The model under review builds one solid part; all positions refer to its coordinate system, in mm. Face numbers are marked on the shaded views. A direction names the side the tool comes from. Give positions to 0.01 mm unless a question says otherwise; leave off trailing zeros. Order: outer loops, then holes, each group sorted by start corner. A loop starts at its lowest first (then second) coordinate and runs counter-clockwise, first axis right, second up. Notation, with made-up numbers: (55.5, 77.25) - (82.5, 77.25) arc R34 cw to (82.5, 114.25) - close; hole circle Ø4 at (28.5, 75). An arc over 180 degrees is marked (long way). Put each result on its own line as item: value.
Autodesk Inventor part; units mm, degrees
ref_plane "Work Plane1" through (-126.3, 142.5, 0) normal (0, 1, 0) x (-1, 0, 0)
ref_plane "Work Plane2" through (0, 0, 0) normal (0, 1, 0) x (-1, 0, 0)
ref_plane "Work Plane3" through (0, 0, 0) normal (0, 0, 1) x (1, 0, 0)
sketch "Sketch1" plane through (0, 0, 0) normal (0, 0, 1) x (1, 0, 0)
  line L0 (-126.3, 0) -> (126.3, 0)
  line L1 (126.3, 0) -> (126.3, 142.5)
  line L2 (126.3, 0) -> (268.8, 0) construction
  line L3 (-126.3, 0) -> (-126.3, 142.5)
  point P0 (0, 0)
  dimension "d0" = 252.6
  dimension "d1" = 142.5
  dimension "d2" = 90
  dimension "d3" = 142.5
ref_plane "Work Plane1" through (-126.3, 142.5, 0) normal (0, 1, 0) x (-1, 0, 0)
sketch "Sketch2" plane through (-126.3, 142.5, 0) normal (0, 1, 0) x (-1, 0, 0)
  circle A0 centre (0, 0) radius 10.65
  point P0 (-126.3, 0)
  dimension "d4" = 21.3
sweep "Sweep1" add profiles "Sketch2" path "Sketch1"
ref_plane "Work Plane2" through (0, 0, 0) normal (0, 1, 0) x (-1, 0, 0)
sketch "Sketch3" plane through (0, 0, 0) normal (0, 1, 0) x (-1, 0, 0)
  circle A0 centre (0, 0) radius 11
  dimension "d8" = 22
extrude "Extrusion1" add sketch "Sketch3" along normal blind 17.5
ref_plane "Work Plane3" through (0, 0, 0) normal (0, 0, 1) x (1, 0, 0)
sketch "Sketch4" plane through (0, 0, 0) normal (0, 0, 1) x (1, 0, 0)
  circle A0 centre (0, 12.5) radius 2.5
  point P0 (0, 0)
  dimension "d12" = 5
extrude "Extrusion2" cut sketch "Sketch4" along normal mid plane 100
ref_plane "Work Plane4" through (0, 0, 0) normal (1, 0, 0) x (0, 1, 0)
sketch "Sketch5" plane through (0, 0, 0) normal (1, 0, 0) x (0, 1, 0)
  circle A0 centre (12.5, 0) radius 2.5
  point P0 (0, 0)
  dimension "d16" = 5
extrude "Extrusion3" cut sketch "Sketch5" along normal mid plane 100
sketch "Sketch6" plane through (-126.3, 142.5, 0) normal (0, 1, 0) x (1, 0, 0)
  circle A0 centre (0, 0) radius 10.65
  point P0 (126.3, 0)
sketch "Sketch7" plane through (126.3, 142.5, 0) normal (0, 1, 0) x (1, 0, 0)
  circle A0 centre (0, 0) radius 10.65
  point P0 (-126.3, 0)
ref_plane "Work Plane6" through (126.3, 0, 0) normal (1, 0, 0) x (0, 1, 0)
ref_plane "Work Plane7" through (-126.3, 0, 0) normal (1, 0, 0) x (0, 1, 0)
sketch "Sketch8" plane through (-126.3, 0, 0) normal (1, 0, 0) x (0, 1, 0)
  line L0 (142.5, -10.65) -> (142.5, 10.65)
  circle A0 centre (130, 0) radius 10.65
  point P0 (0, 0)
  point P1 (142.5, 0)
  dimension "d21" = 21.3
extrude "Extrusion4" add sketch "Sketch8" against normal blind 100
sketch "Sketch9" plane through (126.3, 0, 0) normal (1, 0, 0) x (0, 1, 0)
  circle A0 centre (130, 0) radius 10.65
  circle A1 centre (130, 0) radius 10.65
  point P0 (0, 0)
extrude "Extrusion5" add sketch "Sketch9" along normal blind 100
properties part number "hands" material "PVC-Piping"
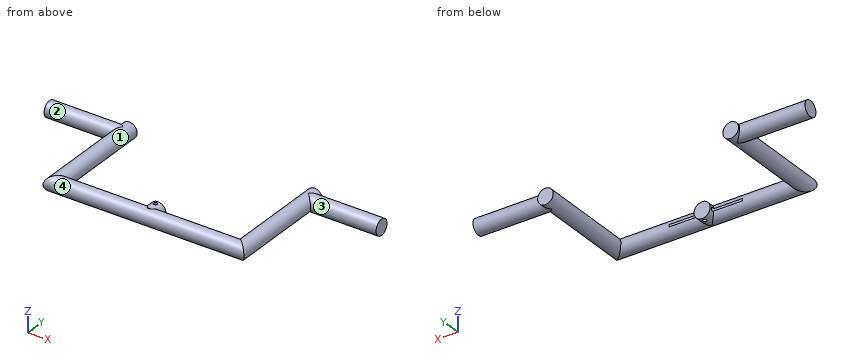
(1) Wall thickness on L1, parallel to X at y = 16.5, z = -1; L2, parallel to X at y = 42, z = 1; L3, parallel to X at y = 12.5, z = 2.75: over which ranges is each line inside the solid? List them lowest first.
The answers:
L1: -136.9 to -115.7, -10.95 to 10.95, 115.7 to 136.9
L2: -136.9 to -115.7, 115.7 to 136.9
L3: -136.59 to -116.01, -10.65 to -2.5, 2.5 to 10.65, 116.01 to 136.59
(2) Take a section at D-D, the plane x = -27. Write out the cut boundary in (y, z), then the cut area to 3 significant figures.
The answers:
outline: (10.54, -1.55) arc R2.5 cw to (10.54, 1.55) arc R10.65 ccw (long way) to start
area: 355 mm^2
(3) The part is to be moulded in two halves that separate along X. For the marked faces 3 and 4, say which applies: pulls with the +X half, pulls with the -X half, needs draft (parallel to the pull), parting line crosses it, or undercut.
The answers:
face 3: needs draft
face 4: undercut
(4) Take a section at B-B, the plane x = 130.5. Write out the cut boundary in (y, z), then the cut area to 3 significant figures.
The answers:
outline: (-4.2, -9.79) - (125.8, -9.79) arc R10.65 ccw to (134.2, -9.79) - (142.5, -9.79) - (142.5, 9.79) - (134.2, 9.79) arc R10.65 ccw to (125.8, 9.79) - (-4.2, 9.79) arc R10.65 ccw to start
area: 2,970 mm^2
(5) For the marked faces 1 and 2, list the 3-axis set-ups (+Z, -Z, +X, -X, +Y, -Y) from which the entire face can be reached by the end or side of a thin tool; tool diameter is ignored.
The answers:
face 1: none
face 2: -X
(6) Clearance check with flat-ended pins moving along their axes: pin 1 Ø5 at (x, z) = (179.5, 7) entering from -Y; pin 2 Ø8 at (y, z) = (69.5, 4) entering from +X; pin 3 Ø2 at (x, z) = (-92, 4.5) entering from +Y; pin 4 Ø6 at (x, y) = (0, 12.5) entering from +Z. State where each tip first meets the part, or that it passes through.
The answers:
pin 1: y = 120.35
pin 2: x = 136.95
pin 3: y = 10.06
pin 4: z = 11
(7) Take a section at C-C, the plane x = -183. Write out the cut boundary in (y, z), then the cut area to 3 significant figures.
The answers:
outline: circle Ø21.3 at (130, 0)
area: 356 mm^2
(8) Take a section at A-A, the plane y = 78. Write out the cut boundary in (x, z), then the cut area to 3 significant figures.
The answers:
outline: circle Ø21.3 at (-126.3, 0); circle Ø21.3 at (126.3, 0)
area: 713 mm^2
